Autodesk Inventor part; units mm, degrees
ref_plane "YZ Plane" through (0, 0, 0) normal (1, 0, 0) x (0, 1, 0)
ref_plane "XZ Plane" through (0, 0, 0) normal (0, 1, 0) x (-1, 0, 0)
ref_plane "XY Plane" through (0, 0, 0) normal (0, 0, 1) x (1, 0, 0)
sketch "hole" plane through (0, 0, 0) normal (0, 0, 1) x (1, 0, 0)
  line L0 (16.5616, -7.6441) -> (20.1684, -7.6441)
  line L1 (20.6764, -8.1521) -> (20.6764, -11.7589)
  line L2 (20.1684, -12.2669) -> (16.5616, -12.2669)
  line L3 (16.0536, -11.7589) -> (16.0536, -8.1521)
  line L4 (16.0536, -7.6441) -> (20.6764, -12.2669) construction
  line L5 (20.6764, -7.6441) -> (16.0536, -12.2669) construction
  arc A0 (20.6764, -8.1521) -> (20.1684, -7.6441) centre (20.1684, -8.1521) ccw
  arc A1 (20.1684, -12.2669) -> (20.6764, -11.7589) centre (20.1684, -11.7589) ccw
  arc A2 (16.0536, -11.7589) -> (16.5616, -12.2669) centre (16.5616, -11.7589) ccw
  arc A3 (16.5616, -7.6441) -> (16.0536, -8.1521) centre (16.5616, -8.1521) ccw
  point P0 (18.365, -9.9555)
  dimension "d6" = 4.6228
  dimension "d7" = 4.6228
  dimension "d8" = 0.508
sketch "main" plane through (0, 0, 0) normal (0, 0, 1) x (1, 0, 0)
  arc A0 (12.865, -9.9555) -> (23.865, -9.9555) centre (18.365, -9.9555) ccw
  line L0 (12.865, 15.4445) -> (12.865, -9.9555)
  line L1 (23.865, -9.9555) -> (23.865, 7.1895)
  circle A1 centre (32.8381, 19.9475) radius 2.0955
  arc A2 (34.1305, 15.3637) -> (31.6462, 24.5584) centre (32.8381, 19.9475) ccw
  arc A3 (16.9885, 20.7695) -> (12.865, 15.4445) centre (18.365, 15.4445) ccw
  line L2 (16.9885, 20.7695) -> (31.6462, 24.5584)
  line L3 (34.1305, 15.3637) -> (28.9468, 13.9022)
  arc A4 (28.9468, 13.9022) -> (23.865, 7.1895) centre (30.8394, 7.1895) ccw
  line L4 (16.5616, -7.6441) -> (20.1684, -7.6441)
  line L5 (20.6764, -8.1521) -> (20.6764, -11.7589)
  line L6 (20.1684, -12.2669) -> (16.5616, -12.2669)
  line L7 (16.0536, -11.7589) -> (16.0536, -8.1521)
  line L8 (16.0536, -7.6441) -> (20.6764, -12.2669) construction
  line L9 (20.6764, -7.6441) -> (16.0536, -12.2669) construction
  arc A5 (20.6764, -8.1521) -> (20.1684, -7.6441) centre (20.1684, -8.1521) ccw
  arc A6 (20.1684, -12.2669) -> (20.6764, -11.7589) centre (20.1684, -11.7589) ccw
  arc A7 (16.0536, -11.7589) -> (16.5616, -12.2669) centre (16.5616, -11.7589) ccw
  arc A8 (16.5616, -7.6441) -> (16.0536, -8.1521) centre (16.5616, -8.1521) ccw
  line L10 (16.5616, 5.0559) -> (20.1684, 5.0559)
  line L11 (20.6764, 4.5479) -> (20.6764, 0.9411)
  line L12 (20.1684, 0.4331) -> (16.5616, 0.4331)
  line L13 (16.0536, 0.9411) -> (16.0536, 4.5479)
  line L14 (16.0536, 5.0559) -> (20.6764, 0.4331) construction
  line L15 (20.6764, 5.0559) -> (16.0536, 0.4331) construction
  arc A9 (20.6764, 4.5479) -> (20.1684, 5.0559) centre (20.1684, 4.5479) ccw
  arc A10 (20.1684, 0.4331) -> (20.6764, 0.9411) centre (20.1684, 0.9411) ccw
  arc A11 (16.0536, 0.9411) -> (16.5616, 0.4331) centre (16.5616, 0.9411) ccw
  arc A12 (16.5616, 5.0559) -> (16.0536, 4.5479) centre (16.5616, 4.5479) ccw
  line L16 (16.5616, 17.7559) -> (20.1684, 17.7559)
  line L17 (20.6764, 17.2479) -> (20.6764, 13.6411)
  line L18 (20.1684, 13.1331) -> (16.5616, 13.1331)
  line L19 (16.0536, 13.6411) -> (16.0536, 17.2479)
  line L20 (16.0536, 17.7559) -> (20.6764, 13.1331) construction
  line L21 (20.6764, 17.7559) -> (16.0536, 13.1331) construction
  arc A13 (20.6764, 17.2479) -> (20.1684, 17.7559) centre (20.1684, 17.2479) ccw
  arc A14 (20.1684, 13.1331) -> (20.6764, 13.6411) centre (20.1684, 13.6411) ccw
  arc A15 (16.0536, 13.6411) -> (16.5616, 13.1331) centre (16.5616, 13.6411) ccw
  arc A16 (16.5616, 17.7559) -> (16.0536, 17.2479) centre (16.5616, 17.2479) ccw
  point P0 (22.8879, 4.6952)
  dimension "d9" = 12.7
  dimension "d10" = 12.7
  dimension "d12" = 17.145
sketch "Sketch1" plane through (0, 0, 0) normal (0, 1, 0) x (-1, 0, 0)
  arc A0 (-5.5, 0) -> (5.5, 0) centre (0, 0) ccw
  line L0 (-5.5, 25.4) -> (-5.5, 0)
  line L1 (5.5, 0) -> (5.5, 17.145)
  circle A1 centre (14.4731, 29.903) radius 2.0955
  arc A2 (15.7655, 25.3192) -> (13.2812, 34.5139) centre (14.4731, 29.903) ccw
  arc A3 (-1.3765, 30.725) -> (-5.5, 25.4) centre (0, 25.4) ccw
  line L2 (-1.3765, 30.725) -> (13.2812, 34.5139)
  line L3 (15.7655, 25.3192) -> (10.5818, 23.8577)
  arc A4 (10.5818, 23.8577) -> (5.5, 17.145) centre (12.4744, 17.145) ccw
  line L4 (-1.8034, 2.3114) -> (1.8034, 2.3114)
  line L5 (2.3114, 1.8034) -> (2.3114, -1.8034)
  line L6 (1.8034, -2.3114) -> (-1.8034, -2.3114)
  line L7 (-2.3114, -1.8034) -> (-2.3114, 1.8034)
  line L8 (-2.3114, 2.3114) -> (2.3114, -2.3114) construction
  line L9 (2.3114, 2.3114) -> (-2.3114, -2.3114) construction
  arc A5 (2.3114, 1.8034) -> (1.8034, 2.3114) centre (1.8034, 1.8034) ccw
  arc A6 (1.8034, -2.3114) -> (2.3114, -1.8034) centre (1.8034, -1.8034) ccw
  arc A7 (-2.3114, -1.8034) -> (-1.8034, -2.3114) centre (-1.8034, -1.8034) ccw
  arc A8 (-1.8034, 2.3114) -> (-2.3114, 1.8034) centre (-1.8034, 1.8034) ccw
  line L10 (-1.8034, 15.0114) -> (1.8034, 15.0114)
  line L11 (2.3114, 14.5034) -> (2.3114, 10.8966)
  line L12 (1.8034, 10.3886) -> (-1.8034, 10.3886)
  line L13 (-2.3114, 10.8966) -> (-2.3114, 14.5034)
  line L14 (-2.3114, 15.0114) -> (2.3114, 10.3886) construction
  line L15 (2.3114, 15.0114) -> (-2.3114, 10.3886) construction
  arc A9 (2.3114, 14.5034) -> (1.8034, 15.0114) centre (1.8034, 14.5034) ccw
  arc A10 (1.8034, 10.3886) -> (2.3114, 10.8966) centre (1.8034, 10.8966) ccw
  arc A11 (-2.3114, 10.8966) -> (-1.8034, 10.3886) centre (-1.8034, 10.8966) ccw
  arc A12 (-1.8034, 15.0114) -> (-2.3114, 14.5034) centre (-1.8034, 14.5034) ccw
  line L16 (-1.8034, 27.7114) -> (1.8034, 27.7114)
  line L17 (2.3114, 27.2034) -> (2.3114, 23.5966)
  line L18 (1.8034, 23.0886) -> (-1.8034, 23.0886)
  line L19 (-2.3114, 23.5966) -> (-2.3114, 27.2034)
  line L20 (-2.3114, 27.7114) -> (2.3114, 23.0886) construction
  line L21 (2.3114, 27.7114) -> (-2.3114, 23.0886) construction
  arc A13 (2.3114, 27.2034) -> (1.8034, 27.7114) centre (1.8034, 27.2034) ccw
  arc A14 (1.8034, 23.0886) -> (2.3114, 23.5966) centre (1.8034, 23.5966) ccw
  arc A15 (-2.3114, 23.5966) -> (-1.8034, 23.0886) centre (-1.8034, 23.5966) ccw
  arc A16 (-1.8034, 27.7114) -> (-2.3114, 27.2034) centre (-1.8034, 27.2034) ccw
extrude "Extrusion1" add sketch "Sketch1" along normal blind 1.5875
properties part number "bent_gusset_improved" material "Acetal Resin, White"
Could you check a few things on this model? Use its own coordinates, in mm. A direction names the side the tool comes from. Coordinates: 2 decimals unless noted, no trailing zeros. Order: outer loops, then holes, each group sorted by start corner. A loop starts at its lowest first (then second) coordinate and runs counter-clockwise, first axis right, second up.
Q1. Which directions (+Z, -Z, +X, -X, +Y, -Y) give clear straight access to the entire face, cutting with the end or side of a thin tool? Please do faces 5 (the flat face through (-5.85, 0.783, 32.593)), 6 (the flat face through (-5.5, 1, 8)), 7 (the flat face through (2.311, 1, 0)).
Q2. Suppose I cut it at D-D on x = 3.5. Please give me the cut outline in (y, z).
Q3. Suppose I cut it at C-C on z = 15.5. Please give me the cut outline in (x, y).
Q4. Please list where these lines run through material, in increasing order: L1, parallel to X at y = 1.15, z = 12.5; L2, parallel to X at y = 1.05, z = 2.5; L3, parallel to Z at x = -14.5, y = 1.45.
Q5. Suppose I cut it at A-A on y = 1.2. Give the number of separate pieces and of enclosed holes in the cut face, and give its area (3 significant figures).
Q6. Will these pins go through, and if not, where does the flat tip stop? pin 1 (0.8 mm diameter, centred on x = -1, y = 0.5, fed in from +Z); pin 2 (0.8 mm diameter, centred on x = 1, y = 1, fed in from +Z); pin 3 (0.5 mm diameter, centred on y = 1, z = -0.5, fed in from -X).
Q7. Suppose I cut it at B-B on x = 0. Please give me the cut outline in (y, z), and give its area (3 significant figures).
Q8. Thinking about a two-plate mould opening in X: for faces 1 (the flat face through (5.5, 1, 13)), 2 (the cylindrical face through (-0.1, 0.8, -5.5)), 3 (the flat face through (2.311, 1, 25)), 4 (the cylindrical face through (-6.876, 0.783, 21.304)), which applies, released by +X, released by -X, zero draft, split by the parting line, or undercut?
Answer:
1. face 5: +Z, +X, +Y, -Y
1. face 6: -Z, -X, +Y, -Y
1. face 7: +Y, -Y
2. outline: (0, -4.24) - (1.59, -4.24) - (1.59, 29.64) - (0, 29.64) - close
3. outline: (-5.5, 0) - (5.5, 0) - (5.5, 1.59) - (-5.5, 1.59) - close
4. L1: x = -5.5 to -2.31, 2.31 to 5.5
4. L2: x = -5.5 to 5.5
4. L3: z = 24.96 to 27.81, 32 to 34.67
5. separate pieces: 1
5. enclosed holes: 4
5. area: 439 mm2
6. pin 1: stops at z = 31.44
6. pin 2: stops at z = 30.93
6. pin 3: stops at x = -5.49
7. outline: (0, -5.5) - (1.59, -5.5) - (1.59, -2.31) - (0, -2.31) - close; (0, 2.31) - (1.59, 2.31) - (1.59, 10.39) - (0, 10.39) - close; (0, 15.01) - (1.59, 15.01) - (1.59, 23.09) - (0, 23.09) - close; (0, 27.71) - (1.59, 27.71) - (1.59, 31.08) - (0, 31.08) - close
7. area: 36.1 mm2
8. face 1: released by +X
8. face 2: split by the parting line
8. face 3: undercut
8. face 4: released by -X
